Can you work these out from the model? Positions are in its coordinate system, mm. A direction names the side the tool comes from. Coordinates: 2 decimals unless noted, no trailing zeros. Write each loop counter-clockwise with the first axis right and the second up, starting at its lowest first coordinate (ties: lowest second). Pieces come first, ordered by that corner, then holes. Notation, with made-up numbers: (16, 69.5) - (55, 69.5) arc R17 cw to (55, 84.5) - close; hole circle Ø6 at (66, -25). An arc over 180 degrees is marked (long way). Use one line per item in the form item = value. Start each with the question number.
(1) If I drill on probe 1 along Y at (x, z) = (21.05, 4.25); probe 2 along X at (y, z) = (-20.5, 5); probe 3 along Y at (x, z) = (-2.5, 2.25), over which ranges is the centre line in solid material (lowest first)? Write a range as from..to.
(2) If we section it at D-D on y = -2: Please give me the cut outline in (x, z).
(3) If we section it at A-A on x = -26.05: Please give me the cut outline in (y, z).
(4) For pin 1 Ø3 at (x, y) = (-26.05, 23.55) entering from +Z, with a flat end and sliding along its axis, tell me the tip position at first contact or that it passes through.
(5) If we section it at C-C on x = 5: Please give me the cut outline in (y, z), then the cut area to 3 significant figures.
(6) If we section it at B-B on z = 4.5: Please give me the cut outline in (x, y).
(7) Thinking about a two-plate mould opening in Y: for faces 1 (the face through (-1, -30, 3)), 2 (the face through (33.5, -23.5, 3.5)), 3 (the face through (16, 7, 0)), which applies, pulls with the +Y half, pulls with the -Y half, needs draft (parallel to the pull), parting line crosses it, or undercut?
(8) On a 3-axis mill with a long thin cutter (end or side, diameter ignored), from which of +Z, -Z, +X, -X, +Y, -Y can I reach the whole of each face in a straight line? I mean faces 4 (the face through (31.5, 20, 3)), 5 (the face through (-37.5, 0, 3)). Say none if no direction works.
```python
from build123d import *

# Parameters (mm, degrees)
SKETCH1_W                  = 75
SKETCH1_H                  = 60
BOSS_EXTRUDE1_DEPTH        = 7
F_5_3_5_3_DIAMETER_HOLE1_D = 5.3
F_10_0_10_DIAMETER_HOLE1_D = 10
SKETCH5_R                  = 19.5
CUT_EXTRUDE1_DEPTH         = 49.53091798
CUT_EXTRUDE2_DEPTH         = 49.53091798


with BuildPart() as part:
    # Sketch1 → Boss-Extrude1 (new body)
    with BuildSketch(Plane.XY):
        Rectangle(SKETCH1_W, SKETCH1_H)
    extrude(amount=BOSS_EXTRUDE1_DEPTH)

    # Ø5.3 (5.3) Diameter Hole1 (through all)
    with Locations(Plane(origin=(21.05, 23.55, 0), x_dir=(-1, 0, 0), z_dir=(0, 0, -1))):
        with Locations((0, 0), (47.1, 0), (47.1, -47.1), (0, -47.1)):
            Hole(F_5_3_5_3_DIAMETER_HOLE1_D / 2)

    # Ø10.0 (10) Diameter Hole1 (through all)
    with Locations(Plane(origin=(-2.5, 0, 0), x_dir=(-1, 0, 0), z_dir=(0, 0, -1))):
        with Locations((0, 0)):
            Hole(F_10_0_10_DIAMETER_HOLE1_D / 2)

    # Sketch5 → Cut-Extrude1 (cut, through all)
    with BuildSketch(Plane.XY.offset(7)):
        with Locations((-2.5, 0)):
            Circle(SKETCH5_R)
    extrude(amount=-CUT_EXTRUDE1_DEPTH, mode=Mode.SUBTRACT)

    # Sketch6 → Cut-Extrude2 (cut, through all)
    with BuildSketch(Plane(origin=(0, 0, 0), x_dir=(-1, 0, 0), z_dir=(0, 0, -1))):
        with BuildLine():
            Line((-35.5, 18.5), (-35.5, 21.5))
            ThreePointArc((-35.5, 21.5), (-33.5, 23.5), (-31.5, 21.5))
            Line((-31.5, 21.5), (-31.5, 18.5))
            ThreePointArc((-31.5, 18.5), (-33.5, 16.5), (-35.5, 18.5))
        make_face()
        with BuildLine():
            Line((-35.5, -18.5), (-35.5, -21.5))
            ThreePointArc((-35.5, -21.5), (-33.5, -23.5), (-31.5, -21.5))
            Line((-31.5, -21.5), (-31.5, -18.5))
            ThreePointArc((-31.5, -18.5), (-33.5, -16.5), (-35.5, -18.5))
        make_face()
    extrude(amount=-CUT_EXTRUDE2_DEPTH, mode=Mode.SUBTRACT)


solid = part.part
```
Reported:
q1.probe_1 = -30..-26.2, -20.9..20.9, 26.2..30
q1.probe_2 = -37.5..31.5, 35.5..37.5
q1.probe_3 = -30..-19.5, 19.5..30
q2.outline = (-37.5, 0) - (-21.9, 0) - (-21.9, 7) - (-37.5, 7) - close; (16.9, 0) - (37.5, 0) - (37.5, 7) - (16.9, 7) - close
q3.outline = (-30, 0) - (-26.2, 0) - (-26.2, 7) - (-30, 7) - close; (-20.9, 0) - (20.9, 0) - (20.9, 7) - (-20.9, 7) - close; (26.2, 0) - (30, 0) - (30, 7) - (26.2, 7) - close
q4.pin_1 = through
q5.outline = (-30, 0) - (-18, 0) - (-18, 7) - (-30, 7) - close; (18, 0) - (30, 0) - (30, 7) - (18, 7) - close
q5.area = 168 mm2
q6.outline = (-37.5, -30) - (37.5, -30) - (37.5, 30) - (-37.5, 30) - close; hole circle Ø5.3 at (-26.05, -23.55); hole circle Ø5.3 at (-26.05, 23.55); hole circle Ø39 at (-2.5, 0); hole circle Ø5.3 at (21.05, -23.55); hole circle Ø5.3 at (21.05, 23.55); hole (31.5, -21.5) arc R2 ccw to (35.5, -21.5) - (35.5, -18.5) arc R2 ccw to (31.5, -18.5) - close; hole (31.5, 18.5) arc R2 ccw to (35.5, 18.5) - (35.5, 21.5) arc R2 ccw to (31.5, 21.5) - close
q7.face_1 = pulls with the -Y half
q7.face_2 = undercut
q7.face_3 = needs draft
q8.face_4 = +Z, -Z
q8.face_5 = +Z, -Z, -X, +Y, -Y
